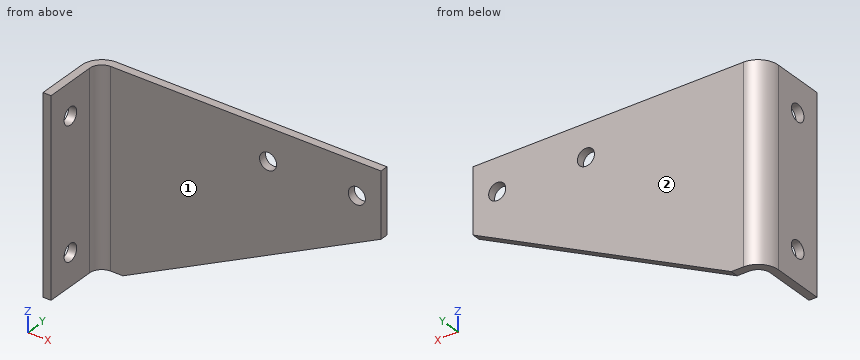
from build123d import *

# Parameters (mm, degrees)
EXTRUDE1_DEPTH         = 127
SKETCH2_R              = 6.731
CUT_CHAMFER_DEPTH      = 508
CUT_CHAMFER_DEPTH_BACK = 58.15
SKETCH3_R              = 6.731
CUT_HOLES_DEPTH        = 229.6
CUT_LH_001_DEPTH       = 58.15


with BuildPart() as part:
    # Sketch1 → Extrude1 (new body, symmetric)
    with BuildSketch(Plane.XY):
        with BuildLine():
            Line((228.6, 0), (15.875, 0))
            ThreePointArc((15.875, 0), (4.649679849, -4.649679849), (0, -15.875))
            Line((0, -15.875), (0, -57.15))
            Line((0, -57.15), (6.35, -57.15))
            Line((6.35, -57.15), (6.35, -15.875))
            ThreePointArc((6.35, -15.875), (9.139807909, -9.139807909), (15.875, -6.35))
            Line((15.875, -6.35), (228.6, -6.35))
            Line((228.6, -6.35), (228.6, 0))
        make_face()
    extrude(amount=EXTRUDE1_DEPTH, both=True)

    # Sketch2 → Cut-Chamfer (cut, two sides)
    with BuildSketch(Plane(origin=(0, 0, 0), x_dir=(1, 0, 0), z_dir=(0, 1, 0))) as cut_chamfer_sk:
        with Locations((209.55, 0)):
            Circle(SKETCH2_R)
        with Locations((139.7, 0)):
            Circle(SKETCH2_R)
        Polygon((25.4, 127), (228.6, 25.4), (228.6, 127), align=None)
        Polygon((25.4, -127), (228.6, -25.4), (228.6, -127), align=None)
    extrude(amount=CUT_CHAMFER_DEPTH, mode=Mode.SUBTRACT)
    extrude(cut_chamfer_sk.sketch, amount=-CUT_CHAMFER_DEPTH_BACK, mode=Mode.SUBTRACT)

    # Sketch3 → Cut-Holes (cut, through all)
    with BuildSketch(Plane(origin=(0, 0, 0), x_dir=(0, 0, -1), z_dir=(1, 0, 0))):
        with Locations((0, -36.5125)):
            Circle(SKETCH3_R)
        with Locations((101.6, -36.5125)):
            Circle(SKETCH3_R)
        with Locations((0, -150.8125)):
            Circle(SKETCH3_R)
        with Locations((101.6, -150.8125)):
            Circle(SKETCH3_R)
        with Locations((-101.6, -36.5125)):
            Circle(SKETCH3_R)
        with Locations((-101.6, -150.8125)):
            Circle(SKETCH3_R)
    extrude(amount=CUT_HOLES_DEPTH, mode=Mode.SUBTRACT)

    # Sketch5 → Cut LH -001 (cut, through all)
    with BuildSketch(Plane(origin=(0, 0, 0), x_dir=(1, 0, 0), z_dir=(0, 1, 0))):
        Polygon((-579.123087515, -25.4), (-7.348788452, -25.4), (228.6, -25.4), (800.374299063, -25.4), (800.374299063, -1168.948598126), (-579.123087515, -1168.948598126), align=None)
    extrude(amount=-CUT_LH_001_DEPTH, mode=Mode.SUBTRACT)


solid = part.part
Could you check a few things on this model? Use its own coordinates, in mm. Face numbers are marked on the shaded views. A direction names the side the tool comes from. Give positions to 0.01 mm unless a question says otherwise; leave off trailing zeros. Order: outer loops, then holes, each group sorted by start corner. A loop starts at its lowest first (then second) coordinate and runs counter-clockwise, first axis right, second up. Notation, with made-up numbers: (53, -14) - (101, -14) arc R14 ccw to (101, 2) - close; hole circle Ø11 at (-1, 40.5). An arc over 180 degrees is marked (long way). Return JSON: item names as keys, results as strings. Group by question number.
Q1. Which directions (+Z, -Z, +X, -X, +Y, -Y) give clear straight access to the entire face, cutting with the end or side of a thin tool? Please do the marked faces 1 and 2.
Q2. Please list where these lines run through material, in increasing order: line 1 along X through (y, z) = (-2, 0); line 2 along X through (y, z) = (-4, 0); line 3 along Y through (x, z) = (183.5, 13). Write a range as [from, to].
Q3. Suppose I cut it at C-C, the plane x = 139.7. Please give me the cut outline in (y, z).
Q4. Will these pins go through, and if not, where does the flat tip stop? pin 1 Ø10 at (y, z) = (-43.5, -17) entering from +X; pin 2 Ø12 at (x, z) = (185, -53) entering from -Y; pin 3 Ø17.5 at (x, z) = (209.55, 0) entering from +Y.
Q5. Suppose I cut it at A-A, the plane z = 0. State how many separate pieces and enclosed holes the cut face has, and give its area (3 significant figures).
Q6. Suppose I cut it at D-D, the plane z = -60. Please give me the cut outline in (x, y) (3 decimals), and give its area (3 significant figures).
Resolved:
{
 "1": {"face 1": "+Z, -Z, +X, -Y", "face 2": "+Z, -Z, +X, -X, +Y"},
 "2": {"line 1": "x = [8.16, 132.97], [146.43, 202.82], [216.28, 228.6]", "line 2": "x = [5.34, 132.97], [146.43, 202.82], [216.28, 228.6]", "line 3": "y = [-6.35, 0]"},
 "3": {"outline": "(-6.35, -69.85) - (0, -69.85) - (0, -6.73) - (-6.35, -6.73) - close; (-6.35, 6.73) - (0, 6.73) - (0, 25.4) - (-6.35, 25.4) - close"},
 "4": {"pin 1": "stops at x = 6.35", "pin 2": "stops at y = -6.35", "pin 3": "stops at y = 0"},
 "5": {"separate pieces": "4", "enclosed holes": "0", "area": "1,480 mm2"},
 "6": {"outline": "(0, -57.15) - (6.35, -57.15) - (6.35, -15.875) arc R9.525 cw to (15.875, -6.35) - (159.4, -6.35) - (159.4, 0) - (15.875, 0) arc R15.875 ccw to (0, -15.875) - close", "area": "1,300 mm2"}
}
